from build123d import *

# Parameters (mm, degrees)
SKETCH1_W           = 44
SKETCH1_H           = 44
BOSS_EXTRUDE1_DEPTH = 10
BOSS_EXTRUDE2_DEPTH = 12.7
SKETCH3_R           = 2.6
CUT_EXTRUDE1_DEPTH  = 70.714345726
SKETCH4_R           = 4.275
CUT_EXTRUDE2_DEPTH  = 72.750191637
FILLET1_R           = 3
FILLET2_R           = 5
FILLET3_R           = 0.5
FILLET4_R           = 2


with BuildPart() as part:
    # Sketch1 → Boss-Extrude1 (new body)
    with BuildSketch(Plane.XY):
        Rectangle(SKETCH1_W, SKETCH1_H)
        with BuildLine():
            Line((7, 12), (-7, 12))
            ThreePointArc((-7, 12), (-10.535533906, 10.535533906), (-12, 7))
            Line((-12, 7), (-12, -7))
            ThreePointArc((-12, -7), (-10.535533906, -10.535533906), (-7, -12))
            Line((-7, -12), (7, -12))
            ThreePointArc((7, -12), (10.535533906, -10.535533906), (12, -7))
            Line((12, -7), (12, 7))
            ThreePointArc((12, 7), (10.535533906, 10.535533906), (7, 12))
        make_face(mode=Mode.SUBTRACT)
        with BuildLine():
            Line((-19, 17.2), (-12, 17.2))
            ThreePointArc((-12, 17.2), (-10.25, 15.45), (-12, 13.7))
            Line((-12, 13.7), (-19, 13.7))
            ThreePointArc((-19, 13.7), (-20.75, 15.45), (-19, 17.2))
        make_face(mode=Mode.SUBTRACT)
        with BuildLine():
            Line((-19, -17.2), (-12, -17.2))
            ThreePointArc((-12, -17.2), (-10.25, -15.45), (-12, -13.7))
            Line((-12, -13.7), (-19, -13.7))
            ThreePointArc((-19, -13.7), (-20.75, -15.45), (-19, -17.2))
        make_face(mode=Mode.SUBTRACT)
        with BuildLine():
            Line((12, 17.2), (19, 17.2))
            ThreePointArc((19, 17.2), (20.75, 15.45), (19, 13.7))
            Line((19, 13.7), (12, 13.7))
            ThreePointArc((12, 13.7), (10.25, 15.45), (12, 17.2))
        make_face(mode=Mode.SUBTRACT)
        with BuildLine():
            Line((12, -13.7), (19, -13.7))
            ThreePointArc((19, -13.7), (20.75, -15.45), (19, -17.2))
            Line((19, -17.2), (12, -17.2))
            ThreePointArc((12, -17.2), (10.25, -15.45), (12, -13.7))
        make_face(mode=Mode.SUBTRACT)
    extrude(amount=BOSS_EXTRUDE1_DEPTH)

    # Sketch2 → Boss-Extrude2 (add)
    with BuildSketch(Plane(origin=(22, 0, 0), x_dir=(0, 0, -1), z_dir=(1, 0, 0))):
        Polygon((5, 12), (-50, 12), (-50, 16), (-50, 22), (5, 22), align=None)
    boss_extrude2 = extrude(amount=BOSS_EXTRUDE2_DEPTH)

    # Sketch3 → Cut-Extrude1 (cut, through all)
    with BuildSketch(Plane.XZ.offset(-12)):
        with Locations((28.6, 42)):
            Circle(SKETCH3_R)
        with Locations((28.6, 16)):
            Circle(SKETCH3_R)
    cut_extrude1 = extrude(amount=-CUT_EXTRUDE1_DEPTH, mode=Mode.SUBTRACT)

    # Sketch4 → Cut-Extrude2 (cut, through all)
    with BuildSketch(Plane(origin=(0, 16, 0), x_dir=(-1, 0, 0), z_dir=(0, -1, 0))):
        with Locations(Location((-28.6, -16, 0), (0, 0, 180))):
            Circle(SKETCH4_R)
        with Locations(Location((-28.6, -42, 0), (0, 0, 180))):
            Circle(SKETCH4_R)
    cut_extrude2 = extrude(amount=-CUT_EXTRUDE2_DEPTH, mode=Mode.SUBTRACT)

    # Mirror1: Boss-Extrude2, Cut-Extrude1, Cut-Extrude2 across plane
    add(boss_extrude2.mirror(Plane(origin=(0, 0, 0), x_dir=(0, 0, 1), z_dir=(1, 0, 0))))
    add(cut_extrude1.mirror(Plane(origin=(0, 0, 0), x_dir=(0, 0, 1), z_dir=(1, 0, 0))), mode=Mode.SUBTRACT)
    add(cut_extrude2.mirror(Plane(origin=(0, 0, 0), x_dir=(0, 0, 1), z_dir=(1, 0, 0))), mode=Mode.SUBTRACT)

    # Fillet1
    fillet1_edges = [part.edges().sort_by_distance(p)[0] for p in [
        (34.7, 17, -5),
        (34.7, 17, 50),
        (-34.7, 17, -5),
        (-34.7, 17, 50),
        (-22, 17, 50),
        (22, 17, 50),
    ]]
    fillet(fillet1_edges, radius=FILLET1_R)

    # Fillet2
    fillet2_edges = [part.edges().sort_by_distance(p)[0] for p in [
        (22, -22, 5),
        (-22, -22, 5),
    ]]
    fillet(fillet2_edges, radius=FILLET2_R)

    # Fillet3
    fillet3_edges = [part.edges().sort_by_distance(p)[0] for p in [
        (-22, 17, 10),
        (22, 17, 10),
    ]]
    fillet(fillet3_edges, radius=FILLET3_R)

    # Fillet4
    fillet4_edges = [part.edges().sort_by_distance(p)[0] for p in [
        (-22, 17, -5),
        (22, 17, -5),
    ]]
    fillet(fillet4_edges, radius=FILLET4_R)


solid = part.part
Verification items for the finished model (mm, model axes). A direction names the side the tool comes from. Round coordinates to 2 decimals unless told otherwise and drop trailing zeros. Loops run counter-clockwise (first coordinate to the right, second up) from the corner with the lowest first, then second, coordinate; pieces in that order, holes last. Notation, with made-up numbers: (-21.5, 15.5) - (30.5, 15.5) arc R29 cw to (30.5, 42.5) - close; hole circle Ø10 at (24.25, 14). An arc over 180 degrees is marked (long way). Use a Markdown table: item, result. Add a question column.
1. Section check B-B, the plane z = 16. Record the boundary of the cut face in (x, y) (3 decimals), plus the area to 3 significant figures.
2. Access from +Z, -Z, +X, -X, +Y, -Y to the whole of each face (thin tool, end or side, straight path). Record for faces 1 (the face through (-28, 17, 50)), 2 (the face through (22, -3, 5)), 3 (the face through (-10.25, -15.49, 4.93)), 4 (the face through (32.68, 18.96, 43.28)), 5 (the face through (22, 17, -2)).
3. Release check for a two-part mould opening along Y. For faces 6 (the face through (-15, -13.7, 5)), 7 (the face through (0, -22, 5)), 8 (the face through (-28, 17, -5)) record: released by +Y, released by -Y, zero draft, split by the parting line, or undercut.
4. Section check D-D, the plane z = 23. Record the boundary of the cut face in (x, y).
5. Section check A-A, the plane x = -16. Record the boundary of the cut face in (y, z), plus the area to 3 significant figures.
6. Thickness scan on probe 1 along Z at (x, y) = (-28.6, 13.4); probe 2 along Y at (x, z) = (4, 1.5); probe 3 along Z at (x, y) = (-28.6, 18) (3 decimals). Record the ranges inside material, lowest first. Write a range as [from, to].
7. Section check C-C, the plane y = -3. Record the boundary of the cut face in (x, z), plus the area to 3 significant figures.
8. Gauge pin test, flat ends, axial feed: pin 1 (3 mm diameter, centred on x = -7.5, y = -12, fed in from +Z); pin 2 (1.5 mm diameter, centred on x = -18.5, y = -3.5, fed in from -Z); pin 3 (5 mm diameter, centred on y = -5, z = 3.5, fed in from +X). Record the tip position at first contact, or that the pin passes through.
Checks:
| question | item | result |
|---|---|---|
| 1 | outline | (-34.7, 12) - (-31.2, 12) - (-31.2, 16) - (-32.875, 16) - (-32.875, 22) - (-34.7, 22) - close; (-26, 12) - (-22, 12) - (-22, 22) - (-24.325, 22) - (-24.325, 16) - (-26, 16) - close; (22, 12) - (26, 12) - (26, 16) - (24.325, 16) - (24.325, 22) - (22, 22) - close; (31.2, 12) - (34.7, 12) - (34.7, 22) - (32.875, 22) - (32.875, 16) - (31.2, 16) - close |
| 1 | area | 110 mm^2 |
| 2 | face 1 | +Z, +X, -X, +Y, -Y |
| 2 | face 2 | +Z, -Z, +X, -Y |
| 2 | face 3 | +Z, -Z |
| 2 | face 4 | +Y |
| 2 | face 5 | -Z, +Y, -Y |
| 3 | face 6 | undercut |
| 3 | face 7 | released by -Y |
| 3 | face 8 | zero draft |
| 4 | outline | (-34.7, 12) - (-22, 12) - (-22, 22) - (-34.7, 22) - close; (22, 12) - (34.7, 12) - (34.7, 22) - (22, 22) - close |
| 5 | outline | (-22, 0) - (-17.2, 0) - (-17.2, 10) - (-22, 10) - close; (-13.7, 0) - (13.7, 0) - (13.7, 10) - (-13.7, 10) - close; (17.2, 0) - (22, 0) - (22, 10) - (17.2, 10) - close |
| 5 | area | 370 mm^2 |
| 6 | probe 1 | z = [-5, 13.4], [18.6, 39.4], [44.6, 50] |
| 6 | probe 2 | y = [-22, -12], [12, 22] |
| 6 | probe 3 | z = [-5, 11.725], [20.275, 37.725], [46.275, 50] |
| 7 | outline | (-22, 0) - (-12, 0) - (-12, 10) - (-22, 10) - close; (12, 0) - (22, 0) - (22, 10) - (12, 10) - close |
| 7 | area | 200 mm^2 |
| 8 | pin 1 | stops at z = 10 |
| 8 | pin 2 | stops at z = 0 |
| 8 | pin 3 | stops at x = 22 |
